Geometry check sheet. Reference: the model listing, model coordinates, mm. Face numbers are marked on the shaded views. A direction names the side the tool comes from. Round coordinates to 2 decimals unless told otherwise and drop trailing zeros. Loops run counter-clockwise (first coordinate to the right, second up) from the corner with the lowest first, then second, coordinate; pieces in that order, holes last. Notation, with made-up numbers: (-32, 12.25) -> (6, 12.25) arc R17 ccw to (6, 24.25) -> close; hole circle Ø3 at (-28, -19). An arc over 180 degrees is marked (long way). Use a Markdown table: item, result. Add a question column.
Q1. Gauge pin test, flat ends, axial feed: P1, Ø10, axis at x = 15, y = 36, coming from the +Z side; P2, Ø3, axis at x = 23, z = -6.5, coming from the -Y side (3 decimals); P3, Ø5, axis at y = 14, z = -9.5, coming from the -X side; P4, Ø17, axis at x = 20.625, y = 20.625, coming from the +Z side. Record the tip position at first contact, or that the pin passes through.
Q2. Set-up check for the marked faces 1, 2 and 3: record each of +Z, -Z, +X, -X, +Y, -Y from which the full face is reachable in a straight line by a thin tool's end or side.
Q3. Release check for a two-part mould opening along X. For the marked faces 4, 5 and 6 record: released by +X, released by -X, zero draft, split by the parting line, or undercut.
Q4. Material ranges on L1, parallel to Y at x = 21, z = 5.5; L2, parallel to Z at x = 12, y = 18; L3, parallel to Z at x = 37, y = 9.5, recorded low to high.
Q5. Sectioned sample at B-B, the plane x = 4. Enter the section's corners in (y, z), then the cut area to 3 significant figures.
Q6. Sectioned sample at D-D, the plane z = -6. Enter the section's corners in (x, y) (3 decimals).
Q7. Sectioned sample at A-A, the plane z = 8. Enter the section's corners in (x, y) (3 decimals), then the cut area to 3 significant figures.
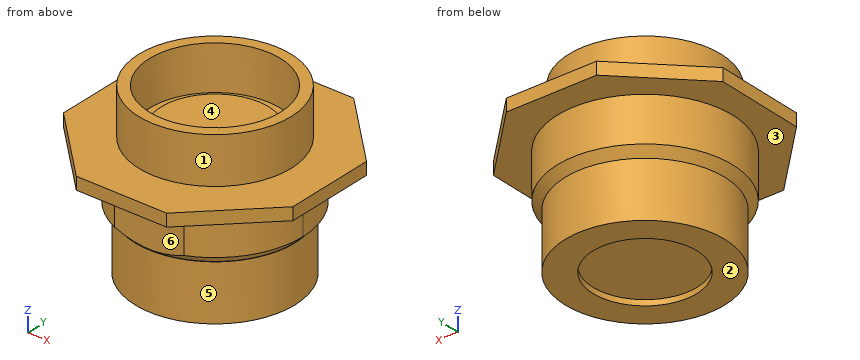
```python
from build123d import *

# Parameters (mm, degrees)
F1_DEPTH    = 2.25
F2_R        = 13.715
F3_DEPTH    = 10.6
F5_DEPTH    = 9.5
F6_T2_ANGLE = 280.2692951884
F6_T4_ANGLE = 100.1752461875
F7_R        = 14.4
F8_DEPTH    = 10
F9_R        = 11.8
F10_DEPTH   = 7
F11_R       = 11.8
F11_R_2     = 9.6734059383
F12_DEPTH   = 8
F13_R       = 9.375
F14_DEPTH   = 1


# Not quite as in the source:
# - a fillet or chamfer that OpenCascade refuses, or shapes differently, is made with other operations: its cross-section is extruded or revolved along the edge and cut away or added


with BuildPart() as f1:
    # F0 (on Top) → F1 (new body)
    with BuildSketch(Plane.XY):
        Polygon((0, 12.5), (12.5, 0), (28.75, 0), (41.25, 12.5), (41.25, 28.75), (28.75, 41.25), (12.5, 41.25), (0, 28.75), align=None)
    extrude(amount=F1_DEPTH)

    # F2 (on Top) → F3 (join)
    with BuildSketch(Plane.XY):
        with Locations((20.625, 20.625)):
            Circle(F2_R)
    extrude(amount=F3_DEPTH)

    # F4 (on face) → F5 (join)
    with BuildSketch(Plane(origin=(0, 0, 0), x_dir=(1, 0, 0), z_dir=(0, 0, -1))):
        with BuildLine():
            ThreePointArc((14.3488546862, -6.125), (11.9509898535, -33.8311178239), (36.425, -20.625))
            ThreePointArc((36.425, -20.625), (33.8311178239, -11.9509898535), (26.9011453138, -6.125))
            Line((26.9011453138, -6.125), (14.3488546862, -6.125))
        make_face()
    extrude(amount=F5_DEPTH)

    # F6: chamfer of 1.5 on 2 edges, made by hand

    # F6_s1 → F6_t2 (revolve, cut)
    with BuildSketch(Plane(origin=(23.5875160096, 4.2735214072, 0), x_dir=(0, 0, 1), z_dir=(0.9839807168, 0.1782749254, 0))):
        with BuildLine():
            Line((-7.9575735931, -0.7752555397), (-9.5424264069, -2.3601083535))
            Line((-9.5424264069, -2.3601083535), (-9.5724264069, -2.3601083535))
            ThreePointArc((-9.5724264069, -2.3601083535), (-9.53, -1.58889515), (-9.53, -0.8176819466))
            Line((-9.53, -0.8176819466), (-9.5, -0.7876819466))
            ThreePointArc((-9.5, -0.7876819466), (-8.7287867966, -0.7876819466), (-7.9575735931, -0.7452555397))
            Line((-7.9575735931, -0.7452555397), (-7.9575735931, -0.7752555397))
        make_face()
    revolve(axis=Axis((20.625, 20.625, -9.5), (0, 0, -1)), revolution_arc=F6_T2_ANGLE, mode=Mode.SUBTRACT)

    # F6_s3 → F6_t4 (revolve, cut)
    with BuildSketch(Plane.XZ.offset(-20.625)):
        with BuildLine():
            Line((36.4674264069, -7.9575735931), (34.8825735931, -9.5424264069))
            Line((34.8825735931, -9.5424264069), (34.8825735931, -9.5724264069))
            ThreePointArc((34.8825735931, -9.5724264069), (35.6537867966, -9.53), (36.425, -9.53))
            Line((36.425, -9.53), (36.455, -9.5))
            ThreePointArc((36.455, -9.5), (36.455, -8.7287867966), (36.4974264069, -7.9575735931))
            Line((36.4974264069, -7.9575735931), (36.4674264069, -7.9575735931))
        make_face()
    revolve(axis=Axis((20.625, 20.625, -9.5), (0, 0, -1)), revolution_arc=F6_T4_ANGLE, mode=Mode.SUBTRACT)

    # F7 (on face) → F8 (join)
    with BuildSketch(Plane(origin=(0, 0, -9.5), x_dir=(1, 0, 0), z_dir=(0, 0, -1))):
        with Locations((20.625, -20.625)):
            Circle(F7_R)
    extrude(amount=F8_DEPTH)

    # F9 (on face) → F10 (cut)
    with BuildSketch(Plane.XY.offset(10.6)):
        with Locations((20.625, 20.625)):
            Circle(F9_R)
    extrude(amount=-F10_DEPTH, mode=Mode.SUBTRACT)

    # F11 (on face) → F12 (cut)
    with BuildSketch(Plane.XY.offset(10.6)):
        with Locations((20.625, 20.625)):
            Circle(F11_R)
        with Locations((20.625, 20.625)):
            Circle(F11_R_2, mode=Mode.SUBTRACT)
    extrude(amount=-F12_DEPTH, mode=Mode.SUBTRACT)

    # F13 (on face) → F14 (cut)
    with BuildSketch(Plane(origin=(0, 0, -19.5), x_dir=(1, 0, 0), z_dir=(0, 0, -1))):
        with Locations((20.625, -20.625)):
            Circle(F13_R)
    extrude(amount=-F14_DEPTH, mode=Mode.SUBTRACT)


solid = f1.part
```
Values:
| question | item | result |
|---|---|---|
| 1 | P1 | z = 10.6 |
| 1 | P2 | y = 6.125 |
| 1 | P3 | x = 5.52 |
| 1 | P4 | z = 3.6 |
| 2 | face 1 | +Z |
| 2 | face 2 | -Z, +X, -X, +Y, -Y |
| 2 | face 3 | -Z |
| 3 | face 4 | undercut |
| 3 | face 5 | split by the parting line |
| 3 | face 6 | zero draft |
| 4 | L1 | 6.92 to 8.83, 32.42 to 34.33 |
| 4 | L2 | -18.5 to 3.6 |
| 4 | L3 | 0 to 2.25 |
| 5 | outline | (8.5, 0) -> (32.75, 0) -> (32.75, 2.25) -> (8.5, 2.25) -> close |
| 5 | area | 54.6 mm^2 |
| 6 | outline | (14.349, 6.125) -> (26.901, 6.125) arc R15.8 ccw (long way) to start |
| 7 | outline | circle Ø27.43 at (20.625, 20.625); hole circle Ø23.6 at (20.625, 20.625) |
| 7 | area | 154 mm^2 |
